Check sheet for the drawn part. Datum: minimum x, y, z corner. Units: mm. A direction names the side the tool comes from. Give positions to 0.01 mm unless a question says otherwise; leave off trailing zeros. Loops run counter-clockwise (first coordinate to the right, second up) from the corner with the lowest first, then second, coordinate; pieces in that order, holes last. Notation, with made-up numbers: (76, 33.25) - (92, 33.25) arc R17 cw to (92, 54.25) - close; hole circle Ø8 at (22, -8). An arc over 180 degrees is marked (long way). Answer in a Markdown table with one row per item.
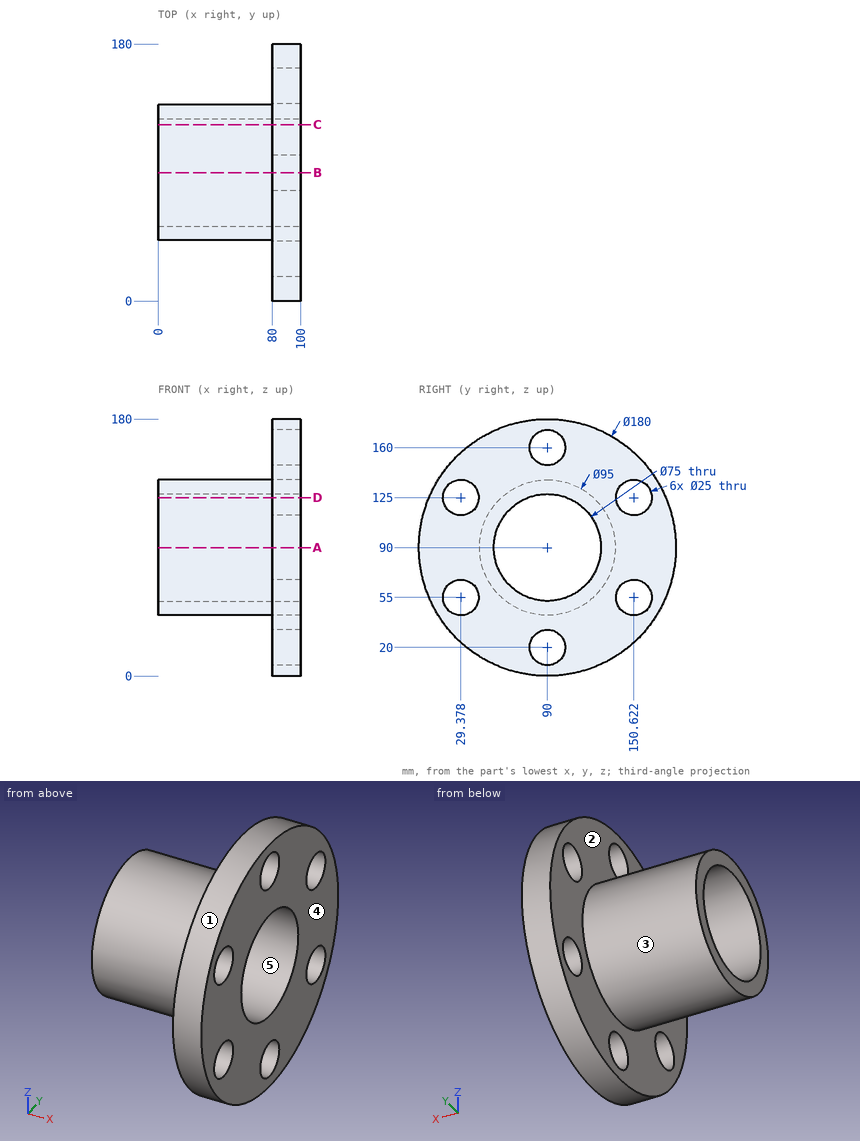
Q1. Sectioned sample at A-A (z = 90). Record the cut outline in (x, y), and give its area (3 significant figures).
Completed:
| item | result |
|---|---|
| outline | (0, 42.5) - (80, 42.5) - (80, 0) - (100, 0) - (100, 52.5) - (0, 52.5) - close; (0, 127.5) - (100, 127.5) - (100, 180) - (80, 180) - (80, 137.5) - (0, 137.5) - close |
| area | 3,700 mm^2 |
Q2. Sectioned sample at C-C (y = 123.5). Record the cut outline in (x, z) (1 decimal), and give its area (3 significant figures).
Completed:
| item | result |
|---|---|
| outline | (0, 56.3) - (80, 56.3) - (80, 6.5) - (100, 6.5) - (100, 73.1) - (0, 73.1) - close; (0, 106.9) - (100, 106.9) - (100, 173.5) - (80, 173.5) - (80, 123.7) - (0, 123.7) - close |
| area | 5,360 mm^2 |
Q3. Draft check along Y on the marked faces 3, 4 and 5. Enter one of: +Y half, -Y half, draft (parallel to the pull), parting line (faces both ways), or undercut.
Completed:
| item | result |
|---|---|
| face 3 | parting line |
| face 4 | draft |
| face 5 | undercut |
Q4. Thickness scan on line 1 (X direction, y = 152.5, z = 90.5); line 2 (Z direction, x = 70.5, y = 89); line 3 (Z direction, x = 18, y = 107.5). Record the ranges inside material, lowest first.
Completed:
| item | result |
|---|---|
| line 1 | 80 to 100 |
| line 2 | 42.51 to 52.51, 127.49 to 137.49 |
| line 3 | 45.84 to 56.83, 123.17 to 134.16 |
Q5. Sectioned sample at D-D (z = 125). Record the cut outline in (x, y), and give its area (3 significant figures).
Completed:
| item | result |
|---|---|
| outline | (0, 57.89) - (80, 57.89) - (80, 41.88) - (100, 41.88) - (100, 76.54) - (0, 76.54) - close; (0, 103.46) - (100, 103.46) - (100, 138.12) - (80, 138.12) - (80, 122.11) - (0, 122.11) - close; (80, 7.08) - (100, 7.08) - (100, 16.88) - (80, 16.88) - close; (80, 163.12) - (100, 163.12) - (100, 172.92) - (80, 172.92) - close |
| area | 4,760 mm^2 |
Q6. Tool access check on the marked faces 1 and 2. Record the directions out of +Z, -Z, +X, -X, +Y, -Y that give a thin tool (end or side, any length) a straight path to the whole face; none if there is none.
Completed:
| item | result |
|---|---|
| face 1 | +X, -X |
| face 2 | -X |
Q7. Go/stop test with flat-tipped pins: P1, Ø22.5, axis at y = 90, z = 20, coming from the -X side; P2, Ø1, axis at x = 32.5, y = 86, coming from the -Z side; P3, Ø1.5, axis at x = 27, y = 51.5, coming from the +Z side; P4, Ø3, axis at x = 82.5, z = 136.5, coming from the -Y side. Record where each tip stops, or that it passes through.
Completed:
| item | result |
|---|---|
| P1 | through |
| P2 | z = 42.63 |
| P3 | z = 118.83 |
| P4 | y = 12.06 |
Q8. Sectioned sample at B-B (y = 90). Record the cut outline in (x, z), and give its area (3 significant figures).
Completed:
| item | result |
|---|---|
| outline | (0, 42.5) - (80, 42.5) - (80, 32.5) - (100, 32.5) - (100, 52.5) - (0, 52.5) - close; (0, 127.5) - (100, 127.5) - (100, 147.5) - (80, 147.5) - (80, 137.5) - (0, 137.5) - close; (80, 0) - (100, 0) - (100, 7.5) - (80, 7.5) - close; (80, 172.5) - (100, 172.5) - (100, 180) - (80, 180) - close |
| area | 2,700 mm^2 |
